For this review, take the finished solid that the model builds, in its own axes (mm). A direction names the side the tool comes from. Coordinates: 2 decimals unless noted, no trailing zeros. Order: outer loops, then holes, each group sorted by start corner. A loop starts at its lowest first (then second) coordinate and runs counter-clockwise, first axis right, second up. Notation, with made-up numbers: M 37,37 L 62,37 A29 ccw 62,66 Z; hole C 57.25,34.25 d8. An arc over 180 degrees is marked long. Use CSV: the item, a comma, the result in double quotes.
```python
from build123d import *

# Parameters (mm, degrees)
SKETCH1_R           = 35
SKETCH1_R_2         = 25
BOSS_EXTRUDE1_DEPTH = 15
BOSS_EXTRUDE2_START = 3
SKETCH2_R           = 45
SKETCH2_R_2         = 25
BOSS_EXTRUDE2_DEPTH = 3
SKETCH3_R           = 1.5
FILLET1_R           = 0.5


with BuildPart() as part:
    # Sketch1 → Boss-Extrude1 (new body)
    with BuildSketch(Plane(origin=(0, 0, 0), x_dir=(0, 1, 0), z_dir=(0, 0, 1))):
        with Locations(Location((0, 0, 0), (0, 0, 270))):
            Circle(SKETCH1_R)
        with Locations(Location((0, 0, 0), (0, 0, 270))):
            Circle(SKETCH1_R_2, mode=Mode.SUBTRACT)
    extrude(amount=-BOSS_EXTRUDE1_DEPTH)

    # Sketch2 → Boss-Extrude2 (add)
    with BuildSketch(Plane.XY.offset(BOSS_EXTRUDE2_START)):
        Circle(SKETCH2_R)
        Circle(SKETCH2_R_2, mode=Mode.SUBTRACT)
    extrude(amount=-BOSS_EXTRUDE2_DEPTH)

    # Sketch3 → Revolve1 (revolve)
    with BuildSketch(Plane.YZ, mode=Mode.PRIVATE) as revolve1_sk:
        with Locations((-35, 3)):
            Circle(SKETCH3_R)
    revolve(revolve1_sk.sketch.rotate(Axis((0, 0, 13.091516213), (0, 0, -1)), 270), axis=Axis((0, 0, 13.091516213), (0, 0, -1)))

    # Fillet1
    fillet1_edges = [part.edges().sort_by_distance(p)[0] for p in [
        (-45, 0, 3),
        (-45, 0, 0),
        (-25, 0, 3),
    ]]
    fillet(fillet1_edges, radius=FILLET1_R)


solid = part.part
```
Item 1: Add section C-C on z = -10.5. State the section outline as (x, y) points, and give its area (3 significant figures).
Solutions:
outline,"C 0,0 d70; hole C 0,0 d50"
area,"1,880 mm^2"
Item 2: Clearance check with flat-ended pins moving along their axes: pin 1 Ø5 at (x, z) = (27.5, -7.5) entering from -Y; pin 2 Ø1.5 at (x, z) = (-8, -7) entering from +Y; pin 3 Ø5 at (y, z) = (-34, -5) entering from -X. State where each tip first meets the part, or that it passes through.
Solutions:
pin 1,"y = -24.49"
pin 2,"y = 34.24"
pin 3,"x = -15.26"
Item 3: For faces 4 (the face through (-27, -23, 0)), 5 (the face through (-24, 8, -15)), list the 3-axis set-ups (+Z, -Z, +X, -X, +Y, -Y) from which the entire face can be reached by the end or side of a thin tool; tool diameter is ignored.
Solutions:
face 4,"-Z"
face 5,"-Z, +X, -X, +Y, -Y"
Item 4: Add section A-A on x = 0. State the section outline as (y, z) points, and give its area (3 significant figures).
Solutions:
outline,"M -45,0.5 A0.5 ccw -44.5,0 L -35,0 L -35,-15 L -25,-15 L -25,2.5 A0.5 ccw -25.5,3 L -33.5,3 A1.5 ccw -36.5,3 L -44.5,3 A0.5 ccw -45,2.5 Z; M 25,-15 L 35,-15 L 35,0 L 44.5,0 A0.5 ccw 45,0.5 L 45,2.5 A0.5 ccw 44.5,3 L 36.5,3 A1.5 ccw 33.5,3 L 25.5,3 A0.5 ccw 25,2.5 Z"
area,"427 mm^2"
Item 5: Draft analysis for pull direction Y (two halves, no side actions). For faces 1 (the face through (-28, -21, -7)), 2 (the face through (-8, -25, 3)), 3 (the face through (-3.5, 36.5, 3)), state which applies: released by +Y, released by -Y, zero draft, split by the parting line, or undercut.
Solutions:
face 1,"split by the parting line"
face 2,"undercut"
face 3,"zero draft"
Item 6: To check wall thickness, follow line 1 along Z through (x, y) = (23, -14); line 2 along Z through (x, y) = (-35.5, -25.5); line 3 along Y through (x, z) = (-17.5, -9.5). State the ranges of each line that lie inside material, in increasing order. Write a range as [from, to].
Solutions:
line 1,"[-15, 3]"
line 2,"[0, 3]"
line 3,"[-30.31, -17.85], [17.85, 30.31]"
